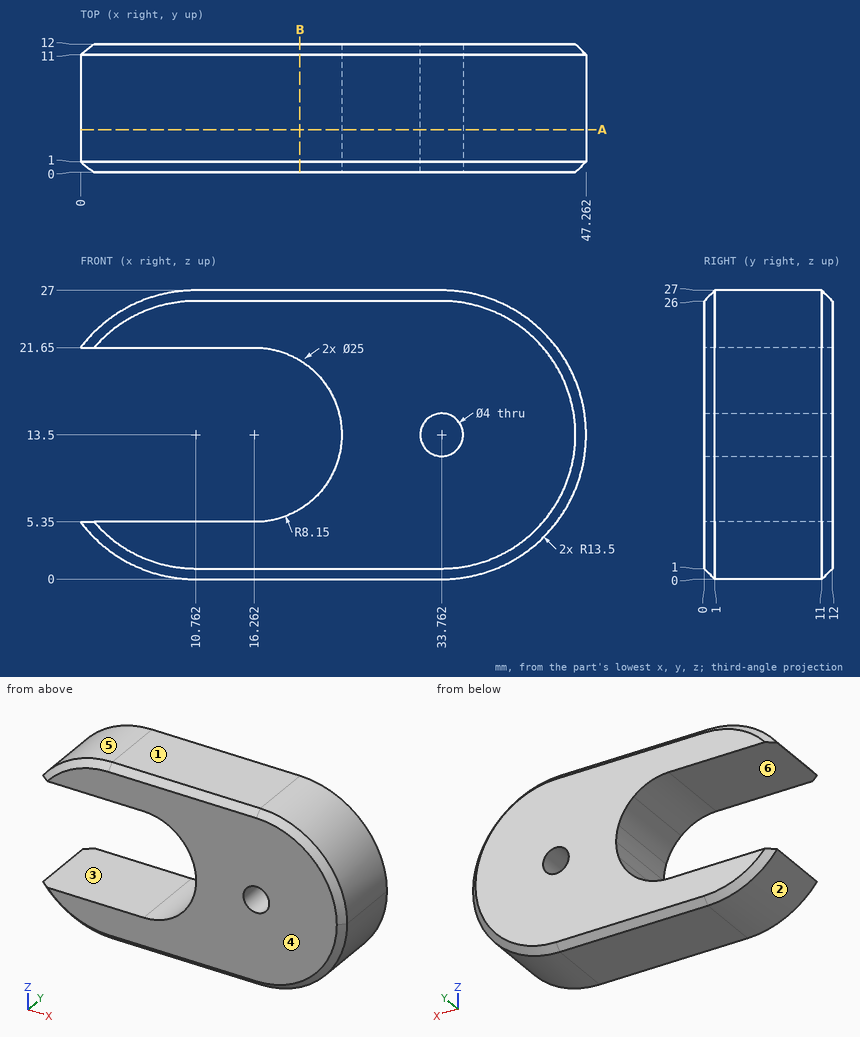
Study the drawing (mm; zero at the part's minimum x, y, z) and answer. A direction names the side the tool comes from. Round coordinates to 2 decimals unless told otherwise and drop trailing zeros. Write each loop counter-clockwise with the first axis right and the second up, starting at its lowest first coordinate (ties: lowest second). Pieces come first, ordered by that corner, then holes.
1) Straight lines are drawn through the part: line 1 (Z direction, x = 16, y = 6); line 2 (Z direction, x = 17, y = 2); line 3 (X direction, y = 2.5, z = 5.25) (1 decimal). For each, find the intervals that lie inside material, in ascending order.
2) A tool of negligible diameter and unlimited length cuts with its end or side. For the marked faces 5 and 6, from which of +Z, -Z, +X, -X, +Y, -Y can it reach the whole face along a straight path? Write none if from no direction.
3) The mould has two halves that part along Z. Classify the marked faces 1, 2, 3 and 4: pulls with the +Z half, pulls with the -Z half, needs draft (parallel to the pull), parting line crosses it, or undercut.
4) A cutting plane is placed at B-B (x = 20.5). Give the vertices of the cut face in (y, z).
5) Given pin 1 Ø1 at (x, y) = (5, 10) entering from +Z; pin 2 Ø3 at (y, z) = (9.5, 22.5) entering from -X, each flat-ended and moving along its own axis, determine where each tip first touches the part or whether it passes through.
6) A cutting plane is placed at A-A (y = 4). Give the vertices of the cut face in (x, z), plus the area to 3 significant figures.
Completed:
1. line 1: z = 0 to 5.35, 21.65 to 27
1. line 2: z = 0 to 5.38, 21.62 to 27
1. line 3: x = 0.1 to 44.4
2. face 5: +Z, -X, +Y, -Y
2. face 6: -X, +Y, -Y
3. face 1: pulls with the +Z half
3. face 2: pulls with the -Z half
3. face 3: undercut
3. face 4: needs draft
4. outline: (0, 1) - (1, 0) - (11, 0) - (12, 1) - (12, 6.54) - (0, 6.54) - close; (0, 20.46) - (12, 20.46) - (12, 26) - (11, 27) - (1, 27) - (0, 26) - close
5. pin 1: stops at z = 25.93
5. pin 2: stops at x = 0
6. outline: (0, 5.35) arc R13.5 ccw to (10.76, 0) - (33.76, 0) arc R13.5 ccw to (33.76, 27) - (10.76, 27) arc R13.5 ccw to (0, 21.65) - (16.26, 21.65) arc R8.15 cw to (16.26, 5.35) - close; hole circle Ø4 at (33.76, 13.5)
6. area: 781 mm2
